For this review, take the finished solid that the model builds, in its own axes (mm). Round coordinates to 2 decimals unless told otherwise and drop trailing zeros. Write each loop counter-clockwise with the first axis right and the second up, starting at its lowest first coordinate (ties: lowest second). Pieces come first, ordered by that corner, then holes. Notation, with made-up numbers: M 8,34.25 L 39,34.25 A28 cw 39,56.25 Z; hole C 30.5,-8.75 d9. An arc over 180 degrees is marked long. Answer in a Markdown table with one row per item.
```python
from build123d import *

# Parameters (mm, degrees)
ESQUISSE1_W                  = 600
ESQUISSE1_H                  = 100
BOSS_EXTRU_1_DEPTH           = 30
ENL_V_MAT_EXTRU_1_DEPTH      = 610.015599143
ENL_V_MAT_EXTRU_1_DEPTH_BACK = 610.015599143
ESQUISSE2_R                  = 38.5


with BuildPart() as part:
    # Esquisse1 → Boss.-Extru.1 (new body)
    with BuildSketch(Plane.XY):
        with Locations((300, 50)):
            Rectangle(ESQUISSE1_W, ESQUISSE1_H)
    extrude(amount=BOSS_EXTRU_1_DEPTH)

    # Esquisse2 → Enlèv. mat.-Extru.1 (cut, two sides: drawn at the far end of the back side and taken through both)
    with BuildSketch(Plane.XY.offset(30).offset(-ENL_V_MAT_EXTRU_1_DEPTH_BACK)):
        with Locations((50, 128.5)):
            Circle(ESQUISSE2_R)
        with Locations((150, 128.5)):
            Circle(ESQUISSE2_R)
        with Locations((250, 128.5)):
            Circle(ESQUISSE2_R)
        with Locations((350, 128.5)):
            Circle(ESQUISSE2_R)
        with Locations((450, 128.5)):
            Circle(ESQUISSE2_R)
        with Locations((550, 128.5)):
            Circle(ESQUISSE2_R)
    extrude(amount=ENL_V_MAT_EXTRU_1_DEPTH + ENL_V_MAT_EXTRU_1_DEPTH_BACK, mode=Mode.SUBTRACT)


solid = part.part
```
Q1. For probe 1 along Y at (x, z) = (448.5, 5.5); probe 2 along Y at (x, z) = (574, 7), list the stretches that pass through material, from the lowest coordinate up.
Found:
| item | result |
|---|---|
| probe 1 | 0 to 90.03 |
| probe 2 | 0 to 98.4 |
Q2. Mouldability with a two-part tool opening along X and no side actions: class faces 1 (the face through (600, 49, 15)), 2 (the face through (50, 90, 15)), 3 (the face through (100, 100, 15)) as +X half, -X half, draft (parallel to the pull), parting line (faces both ways), or undercut.
Found:
| item | result |
|---|---|
| face 1 | +X half |
| face 2 | undercut |
| face 3 | draft |
Q3. Take a section at C-C (x = 346). State the section outline as (y, z) points, then the cut area to 3 significant figures.
Found:
| item | result |
|---|---|
| outline | M 0,0 L 90.21,0 L 90.21,30 L 0,30 Z |
| area | 2,710 mm² |
Q4. Take a section at A-A (z = 24). State the section outline as (x, y) points, then the cut area to 3 significant figures.
Found:
| item | result |
|---|---|
| outline | M 0,0 L 600,0 L 600,100 L 575.88,100 A38.5 cw 524.12,100 L 475.88,100 A38.5 cw 424.12,100 L 375.88,100 A38.5 cw 324.12,100 L 275.88,100 A38.5 cw 224.12,100 L 175.88,100 A38.5 cw 124.12,100 L 75.88,100 A38.5 cw 24.12,100 L 0,100 Z |
| area | 57,900 mm² |
Q5. Take a section at B-B (x = 131.5). State the section outline as (y, z) points.
Found:
| item | result |
|---|---|
| outline | M 0,0 L 94.74,0 L 94.74,30 L 0,30 Z |
